Autodesk Inventor part; units mm, degrees
ref_plane "YZ Plane" through (0, 0, 0) normal (1, 0, 0) x (0, 1, 0)
ref_plane "XZ Plane" through (0, 0, 0) normal (0, 1, 0) x (-1, 0, 0)
ref_plane "XY Plane" through (0, 0, 0) normal (0, 0, 1) x (1, 0, 0)
sketch "Sketch1" plane through (0, 0, 0) normal (0, 0, 1) x (1, 0, 0)
  line L0 (-21, 21) -> (21, 21)
  line L1 (21, 21) -> (21, -21)
  line L2 (21, -21) -> (-21, -21)
  line L3 (-21, -21) -> (-21, 21)
  line L4 (-21, 21) -> (21, -21) construction
  line L5 (21, 21) -> (-21, -21) construction
  circle A0 centre (0, 0) radius 11
  dimension "d0" = 42
  dimension "d1" = 42
  dimension "d2" = 22
extrude "Extrusion1" add sketch "Sketch1" along normal blind 2.5
sketch "Sketch2" plane through (-21, 21, 0) normal (0, 1, 0) x (1, 0, 0)
  line L0 (42, 0) -> (0, 0)
  line L1 (0, 0) -> (0, -2.5)
  line L2 (42, -2.5) -> (0, -2.5)
  line L3 (42, 0) -> (42, -2.5)
  point P0 (21, 0)
extrude "Extrusion2" add sketch "Sketch2" along normal blind 5
sketch "Sketch3" plane through (0, 0, 2.5) normal (0, 0, 1) x (1, 0, 0)
  line L0 (-21, -21) -> (-21, 26)
  line L1 (-21, 26) -> (21, 26)
  line L2 (21, 26) -> (21, 28.5)
  line L3 (21, 28.5) -> (-21, 28.5)
  line L4 (-21, 28.5) -> (-21, 26)
  point P0 (0, 0)
  dimension "d7" = 42
  dimension "d8" = 2.5
extrude "Extrusion3" add sketch "Sketch3" against normal blind 50
properties part number "SOPORTE DE NEMA"
The model under review builds one solid part; all positions refer to its coordinate system, in mm. A direction names the side the tool comes from. Coordinates: 2 decimals unless noted, no trailing zeros. Loops run counter-clockwise (first coordinate to the right, second up) from the corner with the lowest first, then second, coordinate; pieces in that order, holes last.
(1) Wall thickness on L1, parallel to Y at x = 0, z = 1.5; L2, parallel to Y at x = 19, z = -2; L3, parallel to Z at x = -19, y = 25: over which ranges is each line inside the solid? List them lowest first.
Determined:
L1: y = -21 to -11, 11 to 28.5
L2: y = 26 to 28.5
L3: z = 0 to 2.5
(2) Consider section A-A, the plane y = 0. Give the boundary of the cut face in (x, z).
Determined:
outline: (-21, 0) - (-11, 0) - (-11, 2.5) - (-21, 2.5) - close; (11, 0) - (21, 0) - (21, 2.5) - (11, 2.5) - close
(3) Consider section C-C, the plane x = 16. Give the boundary of the cut face in (y, z).
Determined:
outline: (-21, 0) - (26, 0) - (26, -47.5) - (28.5, -47.5) - (28.5, 2.5) - (-21, 2.5) - close
(4) Tool access review of faces 1 (the flat face through (-21, 28, -11)), 2 (the flat face through (0, 13, 0)): name each direction out of +Z, -Z, +X, -X, +Y, -Y from which nothing blocks a thin tool from reaching the whole face with its end or side.
Determined:
face 1: +Z, -Z, -X, +Y, -Y
face 2: -Z, +X, -X, -Y
(5) Consider section D-D, the plane z = -5.5. Give the boundary of the cut face in (x, y).
Determined:
outline: (-21, 26) - (21, 26) - (21, 28.5) - (-21, 28.5) - close
(6) Insertion check: P1, Ø8, axis at x = -16, y = -8, coming from the -Z side; P2, Ø21, axis at x = -5, z = -21.5, coming from the -Y side. Each pin has a flat end and moves straight along its axis. Give the tip position at first contact, or say it passes through.
Determined:
P1: stops at z = 0
P2: stops at y = 26
(7) Draft analysis for pull direction Y (two halves, no side actions). For faces 3 (the flat face through (0, 15, 2.5)), 4 (the cylindrical face through (-2.38, 10.74, 1.23)), 5 (the flat face through (0, 28.5, -22)), state which applies: +Y half, -Y half, draft (parallel to the pull), parting line (faces both ways), or undercut.
Determined:
face 3: draft
face 4: undercut
face 5: +Y half
(8) Consider section B-B, the plane x = 0. Give the boundary of the cut face in (y, z), plus the area to 4 significant figures.
Determined:
outline: (-21, 0) - (-11, 0) - (-11, 2.5) - (-21, 2.5) - close; (11, 0) - (26, 0) - (26, -47.5) - (28.5, -47.5) - (28.5, 2.5) - (11, 2.5) - close
area: 187.5 mm2
